Verification items for the finished model (mm, model axes). A direction names the side the tool comes from. Coordinates: 2 decimals unless noted, no trailing zeros. Order: outer loops, then holes, each group sorted by start corner. A loop starts at its lowest first (then second) coordinate and runs counter-clockwise, first axis right, second up. Notation, with made-up numbers: M 61.25,27.5 L 95.25,27.5 A28 ccw 95.25,59.5 Z; hole C -40,46 d11. An arc over 180 degrees is marked long. Return JSON: item names as keys, results as strings. Group by question number.
1. Set-up check for faces 1 (the flat face through (7, 17, 3)), 2 (the flat face through (21, 7, 0)), 3 (the flat face through (-21, 7, 0)), 4 (the flat face through (-18, 3, -7)): record each of +Z, -Z, +X, -X, +Y, -Y from which the full face is reachable in a straight line by a thin tool's end or side.
2. Section check D-D, the plane y = 14.5. Record the cut outline in (x, z).
3. Section check B-B, the plane z = 0. Record the cut outline in (x, y).
4. Section check A-A, the plane y = 2.75. Record the cut outline in (x, z).
5. Mould release check, pull along X, two halves, no side actions. Record for faces 5 (the cylindrical face through (28, 3, 0)), 6 (the flat face through (-7, 17, 3)), 7 (the flat face through (11, 10, 14)): +X half, -X half, draft (parallel to the pull), parting line (faces both ways), or undercut.
6. Section check C-C, the plane x = 5.5. Record the cut outline in (y, z).
7. Gauge pin test, flat ends, axial feed: pin 1 (11 mm diameter, centred on x = -20, z = 1, fed in from +Y); pin 2 (12 mm diameter, centred on y = 18.5, z = -8.5, fed in from +X); pin 3 (2 mm diameter, centred on x = 18.5, y = 5, fed in from +Z); pin 4 (8 mm diameter, centred on x = -19, y = 22.5, fed in from -Z). Record the tip position at first contact, or that the pin passes through.
8. Material ranges on line 1 along X through (y, z) = (21.25, -2.25); line 2 along X through (y, z) = (16.25, -5.5); line 3 along Z through (x, y) = (16.5, 4.75), recorded low to high.
```python
from build123d import *

# Parameters (mm, degrees)
EXTRUDE_1_DEPTH     = 14
CUT_EXTRUDE_1_DEPTH = 7
EXTRUDE_2_DEPTH     = 7


with BuildPart() as part:
    # 스케치1 → 보스-돌출1 (new body, symmetric)
    with BuildSketch(Plane(origin=(0, 0, 0), x_dir=(0, 0, -1), z_dir=(1, 0, 0))):
        Polygon((14, 0), (-14, 0), (-14, 21), (-7, 28), (14, 28), align=None)
    extrude(amount=EXTRUDE_1_DEPTH, both=True)

    # 스케치2 → 컷-돌출1 (cut, symmetric)
    with BuildSketch(Plane(origin=(0, 0, 0), x_dir=(0, 0, -1), z_dir=(1, 0, 0))):
        Polygon((-14, 0), (14, 28), (-14, 28), align=None)
    extrude(amount=CUT_EXTRUDE_1_DEPTH, both=True, mode=Mode.SUBTRACT)

    # 스케치3 → 보스-돌출2 (add)
    with BuildSketch(Plane(origin=(0, 0, 0), x_dir=(1, 0, 0), z_dir=(0, 1, 0))):
        with BuildLine():
            Line((-21, 7), (-14, 7))
            Line((-14, 7), (-14, -7))
            Line((-14, -7), (-21, -7))
            ThreePointArc((-21, -7), (-28, 0), (-21, 7))
        make_face()
        with BuildLine():
            Line((14, 7), (14, -7))
            Line((14, -7), (21, -7))
            ThreePointArc((21, -7), (28, 0), (21, 7))
            Line((21, 7), (14, 7))
        make_face()
    extrude(amount=EXTRUDE_2_DEPTH)


solid = part.part
```
Answers follow:
{
 "1": {"face 1": "+Z, +Y", "face 2": "+Z, -Z, +X, +Y", "face 3": "+Z, -Z, -X, +Y", "face 4": "-Z, -X, +Y, -Y"},
 "2": {"outline": "M -14,-14 L 14,-14 L 14,14 L 7,14 L 7,-0.5 L -7,-0.5 L -7,14 L -14,14 Z"},
 "3": {"outline": "M -28,0 L 28,0 L 28,7 L 14,7 L 14,28 L 7,28 L 7,14 L -7,14 L -7,28 L -14,28 L -14,7 L -28,7 Z"},
 "4": {"outline": "M -21,-7 L -14,-7 L -14,-14 L 14,-14 L 14,-7 L 21,-7 A7 ccw 21,7 L 14,7 L 14,14 L 7,14 L 7,11.25 L -7,11.25 L -7,14 L -14,14 L -14,7 L -21,7 A7 ccw Z"},
 "5": {"face 5": "+X half", "face 6": "undercut", "face 7": "draft"},
 "6": {"outline": "M 0,-14 L 28,-14 L 0,14 Z"},
 "7": {"pin 1": "y = 7", "pin 2": "x = 14", "pin 3": "z = 7", "pin 4": "through"},
 "8": {"line 1": "-14 to -7, 7 to 14", "line 2": "-14 to 14", "line 3": "-7 to 7"}
}
